Geometry: see drawing. Coordinates: mm, zero at the bounding-box minimum. Coordinates: 2 decimals unless noted, no trailing zeros. Loops run counter-clockwise (first coordinate to the right, second up) from the corner with the lowest first, then second, coordinate; pieces in that order, holes last. Notation, with made-up numbers: (-17.75, 72.5) -> (35.25, 72.5) arc R9 ccw to (35.25, 81.5) -> close; hole circle Ø6 at (4.5, -18.75). An arc over 180 degrees is marked (long way). One line per item, written item: value. Start each with the question number.
Item 1: Contact query for a flat-ended pin moving along its axis: pin 1 Ø6.5 at (x, z) = (7, 6) entering from -Y. Output: stop coordinate, or through.
Item 2: Ray query, probe 1 along Y at (x, z) = (31.5, 9.75); probe 2 along Z at (x, y) = (7, 3); probe 3 along X at (y, z) = (8.75, 6). Return the intervals inside material, ascending. Write a range as from..to.
Item 3: Section query B-B on y = 6. Return loops of the section in (x, z).
Item 4: Section query C-C on x = 7. Return loops of the section in (y, z), then the cut area to 3 significant figures.
Item 5: Mould query, pull axis Z, two halves, no side actions, for the marked faces 1, 2, 3 and 4. Classes: +Z half, -Z half, draft (parallel to the pull), parting line (faces both ways), or undercut.
Item 6: Section query A-A on z = 6. Return loops of the section in (x, y).
Item 7: Section query D-D on y = 3.5. Return loops of the section in (x, z).
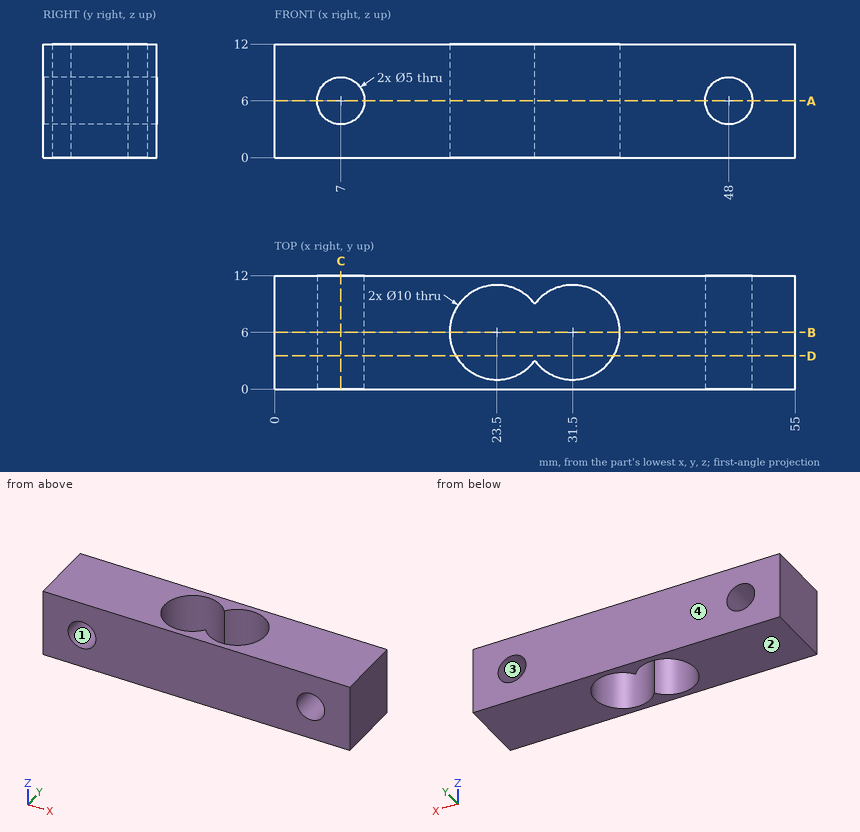
Reply:
1. pin 1: stops at y = 0
2. probe 1: y = 0..1, 11..12
2. probe 2: z = 0..3.5, 8.5..12
2. probe 3: x = 0..4.5, 9.5..19.32, 35.68..45.5, 50.5..55
3. outline: (0, 0) -> (18.5, 0) -> (18.5, 12) -> (0, 12) -> close; (36.5, 0) -> (55, 0) -> (55, 12) -> (36.5, 12) -> close; hole circle Ø5 at (7, 6); hole circle Ø5 at (48, 6)
4. outline: (0, 0) -> (12, 0) -> (12, 3.5) -> (0, 3.5) -> close; (0, 8.5) -> (12, 8.5) -> (12, 12) -> (0, 12) -> close
4. area: 84.0 mm²
5. face 1: undercut
5. face 2: -Z half
5. face 3: undercut
5. face 4: draft
6. outline: (0, 0) -> (4.5, 0) -> (4.5, 12) -> (0, 12) -> close; (9.5, 0) -> (45.5, 0) -> (45.5, 12) -> (9.5, 12) -> close; (50.5, 0) -> (55, 0) -> (55, 12) -> (50.5, 12) -> close; hole (27.5, 3) arc R5 ccw (long way) to (27.5, 9) arc R5 ccw (long way) to start
7. outline: (0, 0) -> (19.17, 0) -> (19.17, 12) -> (0, 12) -> close; (35.83, 0) -> (55, 0) -> (55, 12) -> (35.83, 12) -> close; hole circle Ø5 at (7, 6); hole circle Ø5 at (48, 6)
